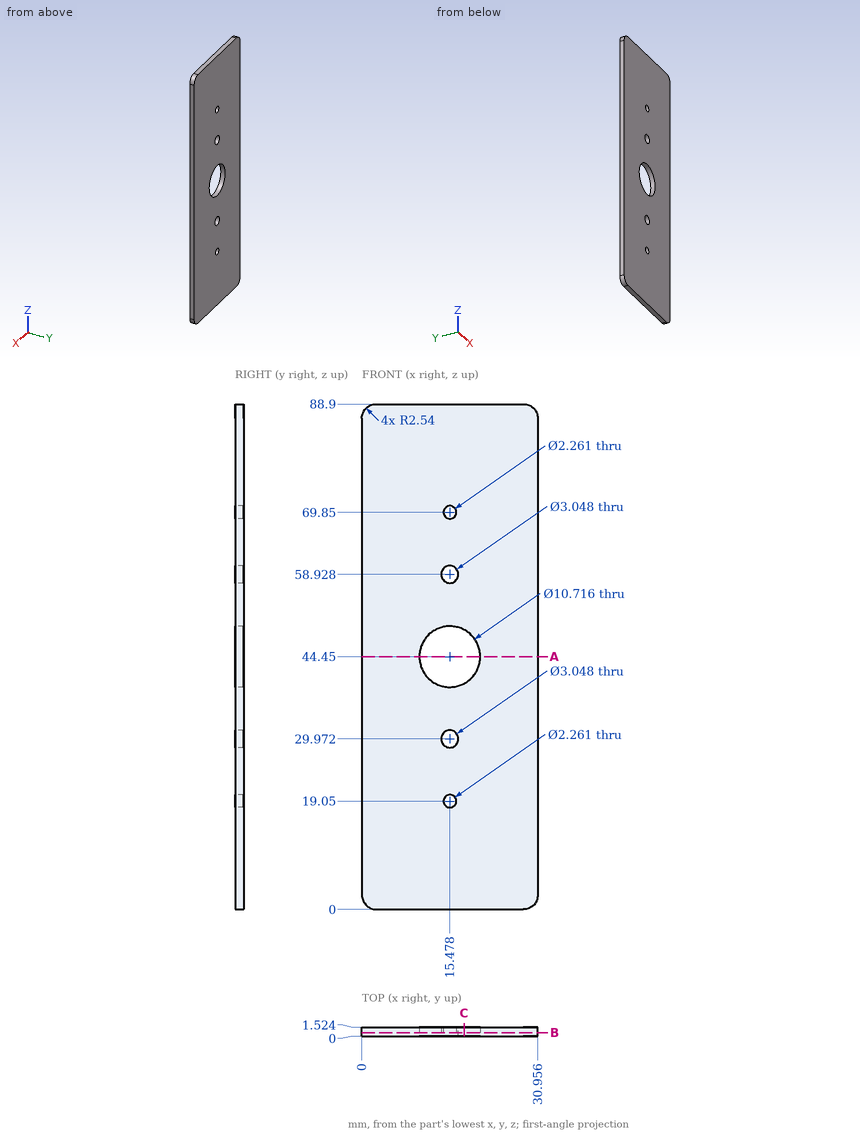
Geometry check sheet. Reference: drawing and pictorial views, mm from the part's lowest x, y, z. Give positions to 0.01 mm unless a question says otherwise; leave off trailing zeros. Order: outer loops, then holes, each group sorted by start corner. A loop starts at its lowest first (then second) coordinate and runs counter-clockwise, first axis right, second up. Notation, with made-up numbers: M 0.5,82 L 42.5,82 A26 ccw 42.5,120 Z; hole C 26.25,15.25 d3. An arc over 180 degrees is marked long. Return JSON: item names as keys, results as strings. Group by question number.
1) Scan lines: line 1 (Z direction, x = 15.5, y = 1.4) (1 decimal); line 2 (X direction, y = 0.75, z = 69.85); line 3 (X direction, y = 0.1, z = 29.5) (1 decimal). Record each from-to range of solid material in increasing order.
2) Section check C-C on x = 18. Record the cut outline in (y, z), and give its area (3 significant figures).
3) Section check B-B on y = 0.6. Record the cut outline in (x, z).
4) Go/stop test with flat-tipped pins: pin 1 Ø3 at (x, z) = (15.48, 69.85) entering from -Y; pin 2 Ø9.5 at (x, z) = (15.48, 44.45) entering from -Y. Record where each tip stops, or that it passes through.
5) Section check A-A on z = 44.45. Record the cut outline in (x, y).
Answer block:
{
 "1": {"line 1": "z = 0 to 17.9, 20.2 to 28.4, 31.5 to 39.1, 49.8 to 57.4, 60.5 to 68.7, 71 to 88.9", "line 2": "x = 0 to 14.35, 16.61 to 30.96", "line 3": "x = 0 to 14, 16.9 to 31"},
 "2": {"outline": "M 0,0 L 1.52,0 L 1.52,39.72 L 0,39.72 Z; M 0,49.18 L 1.52,49.18 L 1.52,88.9 L 0,88.9 Z", "area": "121 mm^2"},
 "3": {"outline": "M 0,2.54 A2.54 ccw 2.54,0 L 28.42,0 A2.54 ccw 30.96,2.54 L 30.96,86.36 A2.54 ccw 28.42,88.9 L 2.54,88.9 A2.54 ccw 0,86.36 Z; hole C 15.48,44.45 d10.72; hole C 15.48,29.97 d3.05; hole C 15.48,58.93 d3.05; hole C 15.48,19.05 d2.26; hole C 15.48,69.85 d2.26"},
 "4": {"pin 1": "stops at y = 0", "pin 2": "passes through"},
 "5": {"outline": "M 0,0 L 10.12,0 L 10.12,1.52 L 0,1.52 Z; M 20.84,0 L 30.96,0 L 30.96,1.52 L 20.84,1.52 Z"}
}
